Build history of the part. All positions in model axes, mm. Round coordinates to 2 decimals unless told otherwise and drop trailing zeros. Loops run counter-clockwise (first coordinate to the right, second up) from the corner with the lowest first, then second, coordinate; pieces in that order, holes last. Notation, with made-up numbers: (28.5, -3) - (82.5, -3) arc R33 cw to (82.5, 25) - close; hole circle Ø9 at (59.25, 79.25). An arc over 180 degrees is marked (long way). Use one line per item in the form item = value. Start each with the question number.
Q1. Saw through at B-B (x = -13). Give the cut face in (y, z).
Q2. Drill centre lines: line 1 (Z direction, x = -6, y = 1.45); line 2 (X direction, y = 1.05, z = -26.5); line 3 (Z direction, x = 5.5, y = 0.75). Where is each one in solid material? Low to high.
Q3. Pin check, flat tips, straight feed: pin 1 (0.6 mm diameter, centred on y = 1.5, z = -8.5, fed in from -X); pin 2 (12 mm diameter, centred on x = 10, z = -13.5, fed in from -Y); pin 3 (1 mm diameter, centred on x = -7.5, z = -20, fed in from +Y); pin 4 (0.8 mm diameter, centred on x = 4, y = 0.5, fed in from -Z). Stop position of each tip, or through.
Q4. Saw through at A-A (x = -2). Give the cut face in (y, z), then the cut area to 3 significant figures.
Q5. Saw through at C-C (y = 1.1). Count the separate pieces of the cut face and the enclosed holes in it, then the cut area to 3 significant figures.
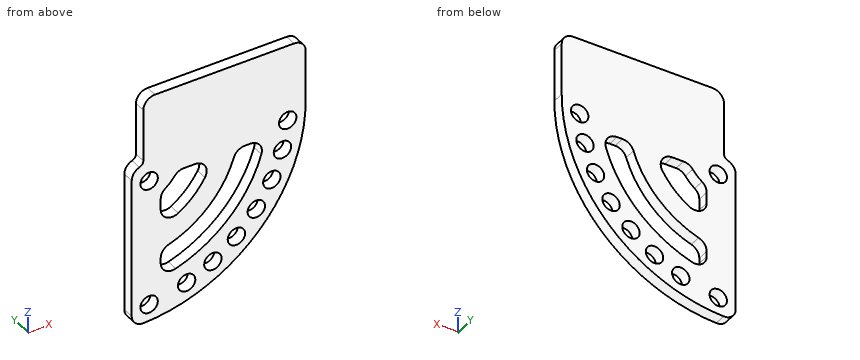
```python
from build123d import *

# Parameters (mm, degrees)
SKETCH_1_R      = 1.5
EXTRUDE_1_DEPTH = 2
FILLET_1_R      = 2


with BuildPart() as part:
    # 草图1 → 凸台-拉伸1 (new body)
    with BuildSketch(Plane(origin=(0, 0, 0), x_dir=(1, 0, 0), z_dir=(0, 1, 0))):
        with BuildLine():
            Line((-11, 0), (0, 0))
            Line((0, 0), (11, 0))
            Line((11, 0), (14, 0))
            Line((14, 0), (14, 11))
            ThreePointArc((14, 11), (5.506096654, 31.506096654), (-15, 40))
            Line((-15, 40), (-16, 40))
            Line((-16, 40), (-16, 12))
            Line((-16, 12), (-15, 12))
            ThreePointArc((-15, 12), (-14.292893219, 11.707106781), (-14, 11))
            Line((-14, 11), (-14, 0))
            Line((-14, 0), (-11, 0))
        make_face()
        with Locations(Location((10.90106215, 13.266049311, 0), (0, 0, 270))):
            Circle(SKETCH_1_R, mode=Mode.SUBTRACT)
        with Locations(Location((9.992804094, 18.166571251, 0), (0, 0, 270))):
            Circle(SKETCH_1_R, mode=Mode.SUBTRACT)
        with Locations(Location((8.166169629, 22.803752993, 0), (0, 0, 270))):
            Circle(SKETCH_1_R, mode=Mode.SUBTRACT)
        with Locations(Location((5.488279594, 27.007198358, 0), (0, 0, 270))):
            Circle(SKETCH_1_R, mode=Mode.SUBTRACT)
        with Locations(Location((2.057534754, 30.622449086, 0), (0, 0, 270))):
            Circle(SKETCH_1_R, mode=Mode.SUBTRACT)
        with Locations(Location((-2, 33.516660498, 0), (0, 0, 270))):
            Circle(SKETCH_1_R, mode=Mode.SUBTRACT)
        with Locations(Location((-6.535227984, 35.583482966, 0), (0, 0, 270))):
            Circle(SKETCH_1_R, mode=Mode.SUBTRACT)
        with Locations(Location((-13, 15, 0), (0, 0, 270))):
            Circle(SKETCH_1_R, mode=Mode.SUBTRACT)
        with Locations(Location((-13, 37, 0), (0, 0, 270))):
            Circle(SKETCH_1_R, mode=Mode.SUBTRACT)
        with BuildLine():
            Line((-11, 24), (-11, 17.92820323))
            ThreePointArc((-11, 17.92820323), (-9.343145751, 16.656854249), (-8.07179677, 15))
            Line((-8.07179677, 15), (-2, 15))
            ThreePointArc((-2, 15), (-5.382307969, 20.617692031), (-11, 24))
        make_face(mode=Mode.SUBTRACT)
        with BuildLine():
            Line((-11, 28), (-11, 33))
            ThreePointArc((-11, 33), (0.811388301, 26.811388301), (7, 15))
            Line((7, 15), (2, 15))
            ThreePointArc((2, 15), (-2.650910965, 23.349089035), (-11, 28))
        make_face(mode=Mode.SUBTRACT)
    extrude(amount=EXTRUDE_1_DEPTH)

    # 圆角1
    fillet_1_edges = [part.edges().sort_by_distance(p)[0] for p in [
        (-14, 1, 0),
        (-16, 1, -12),
        (-16, 1, -40),
        (14, 1, 0),
        (-11, 1, -17.92820323),
        (-8.07179677, 1, -15),
        (-2, 1, -15),
        (-11, 1, -24),
        (7, 1, -15),
        (-11, 1, -28),
        (2, 1, -15),
        (-11, 1, -33),
    ]]
    fillet(fillet_1_edges, radius=FILLET_1_R)


solid = part.part
```
Report:
q1.outline = (0, -39.93) - (2, -39.93) - (2, -38.5) - (0, -38.5) - close; (0, -35.5) - (2, -35.5) - (2, -16.5) - (0, -16.5) - close; (0, -13.5) - (2, -13.5) - (2, -0.27) - (0, -0.27) - close
q2.line_1 = -38.57 to -36.98, -34.18 to -31.47, -25.97 to -21.2, -15 to 0
q2.line_2 = -16 to -6.95, 1.12 to 4.08, 6.9 to 9.51
q2.line_3 = -31.51 to -28.51, -25.51 to -19.93, -15.29 to 0
q3.pin_1 = -14
q3.pin_2 = 0
q3.pin_3 = through
q3.pin_4 = -33.25
q4.outline = (0, -36.92) - (2, -36.92) - (2, -35.02) - (0, -35.02) - close; (0, -32.02) - (2, -32.02) - (2, -29.19) - (0, -29.19) - close; (0, -22.66) - (2, -22.66) - (2, 0) - (0, 0) - close
q4.area = 54.8 mm²
q5.separate_pieces = 1
q5.enclosed_holes = 11
q5.area = 775 mm²
